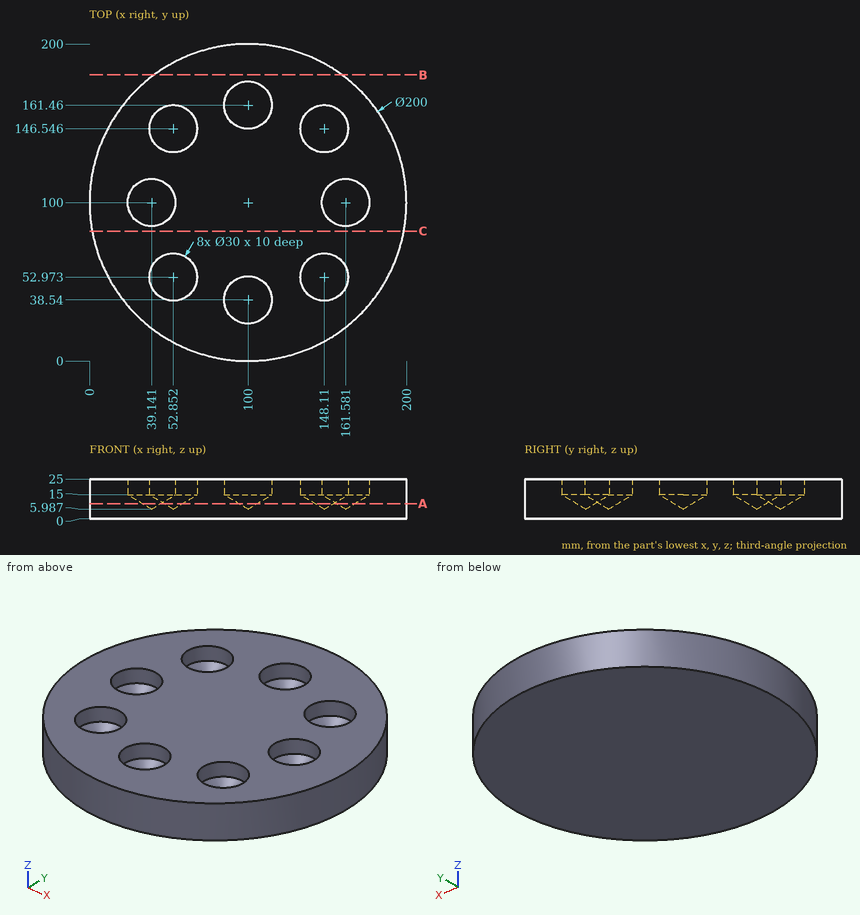
Design review of the part shown in the three views and the two pictorial views. Dimensions are in mm from the part's minimum x, y and z. Round coordinates to 2 decimals unless told otherwise and drop trailing zeros. Loops run counter-clockwise (first coordinate to the right, second up) from the corner with the lowest first, then second, coordinate; pieces in that order, holes last. Notation, with made-up numbers: (39.25, -4) - (58.25, -4) arc R28 cw to (58.25, 29) - close; hole circle Ø3 at (58, 77.25). An arc over 180 degrees is marked (long way). Use one line per item in the form item = value.
1) We need section A-A on z = 9.5. State how many separate pieces and enclosed holes the cut face has, then the cut area to 3 significant figures.
Solutions:
separate_pieces = 1
enclosed_holes = 8
area = 30,600 mm2
2) We need section C-C on y = 82. Write out the cut boundary in (x, z), then the cut area to 3 significant figures.
Solutions:
outline = (1.63, 0) - (198.37, 0) - (198.37, 25) - (1.63, 25) - close
area = 4,920 mm2
3) We need section B-B on y = 180.5. Write out the cut boundary in (x, z), then the cut area to 3 significant figures.
Solutions:
outline = (40.67, 0) - (159.33, 0) - (159.33, 25) - (40.67, 25) - close
area = 2,970 mm2
4) Clearance check with flat-ended pins moving along their axes: P1, Ø1.5, axis at x = 40.5, z = 13, coming from the +Y side; P2, Ø6, axis at y = 33.5, z = 12, coming from the -X side; P3, Ø5, axis at y = 154, z = 10, coming from the -X side; P4, Ø18, axis at x = 148.11, y = 146.55, coming from the -Z side. State where each tip first meets the part, or that it passes through.
Solutions:
P1 = 180.92
P2 = 22.75
P3 = 14.28
P4 = 0
5) Wall thickness on probe 1 along X at (y, z) = (99, 23.5) (1 decimal); probe 2 along Y at (x, z) = (63, 21.25) (1 decimal); probe 3 along Y at (x, z) = (97, 14.25) (1 decimal): over which ranges is each line inside the solid? List them lowest first.
Solutions:
probe_1 = 0 to 24.2, 54.1 to 146.6, 176.5 to 200
probe_2 = 7.1 to 41.9, 64 to 135.5, 157.6 to 192.9
probe_3 = 0 to 25.1, 52 to 148, 174.9 to 200
